Read the model definition and answer for the solid it produces. Units are mm, in the model's axes. A direction names the side the tool comes from. Round coordinates to 2 decimals unless told otherwise and drop trailing zeros.
from build123d import *

# Parameters (mm, degrees)
BOSS_EXTRUDE1_DEPTH     = 15
SKETCH3_W               = 65
SKETCH3_H               = 20
CUT_EXTRUDE2_DEPTH      = 12
CUT_EXTRUDE4_DEPTH      = 52.35659646
M2_TAPPED_HOLE1_D       = 1.6
M2_TAPPED_HOLE1_DEPTH   = 4.519311505
M2_TAPPED_HOLE1_TIP     = 0.480688495
FILLET4_R               = 2.5
SKETCH15_R              = 3
CUT_EXTRUDE10_DEPTH     = 2
CUT_EXTRUDE11_DEPTH     = 8
CUT_EXTRUDE12_DEPTH     = 10
CUT_EXTRUDE13_DEPTH     = 10
SKETCH19_W              = 0.9966679
SKETCH19_H              = 1.5
BOSS_EXTRUDE2_DEPTH     = 20
LPATTERN1_COUNT         = 4
LPATTERN1_PITCH         = 5.5
MIRROR2_COPY_1_SKETCH_W = 0.9966679
MIRROR2_COPY_1_SKETCH_H = 1.5
MIRROR2_COPY_1_DEPTH    = 20
MIRROR2_COPY_2_SKETCH_W = 0.9966679
MIRROR2_COPY_2_SKETCH_H = 1.5
MIRROR2_COPY_2_DEPTH    = 20
MIRROR2_COPY_3_SKETCH_W = 0.9966679
MIRROR2_COPY_3_SKETCH_H = 1.5
MIRROR2_COPY_3_DEPTH    = 20
SKETCH20_W              = 2
SKETCH20_H              = 6
CUT_EXTRUDE14_DEPTH     = 6.5


with BuildPart() as part:
    # Sketch1 → Boss-Extrude1 (new body)
    with BuildSketch(Plane(origin=(0, 0, 0), x_dir=(1, 0, 0), z_dir=(0, 1, 0))):
        Polygon((-47.5, -6.5), (-41.5, -12.5), (41.5, -12.5), (47.5, -6.5), (47.5, 6.5), (41.5, 12.5), (-41.5, 12.5), (-47.5, 6.5), align=None)
    extrude(amount=BOSS_EXTRUDE1_DEPTH)

    # Sketch3 → Cut-Extrude2 (cut)
    with BuildSketch(Plane(origin=(0, 15, 0), x_dir=(1, 0, 0), z_dir=(0, 1, 0))):
        Rectangle(SKETCH3_W, SKETCH3_H)
    extrude(amount=-CUT_EXTRUDE2_DEPTH, mode=Mode.SUBTRACT)

    # Sketch4 → Cut-Extrude4 (cut, through all)
    with BuildSketch(Plane(origin=(0, 15, 0), x_dir=(1, 0, 0), z_dir=(0, 1, 0))):
        with BuildLine():
            Line((41.610912703, 9.560660172), (45.696699141, 5.474873734))
            ThreePointArc((45.696699141, 5.474873734), (45.98959236, 4.767766953), (45.696699141, 4.060660172))
            Line((45.696699141, 4.060660172), (43.575378798, 1.939339828))
            ThreePointArc((43.575378798, 1.939339828), (42.868272016, 1.646446609), (42.161165235, 1.939339828))
            Line((42.161165235, 1.939339828), (38.075378798, 6.025126266))
            ThreePointArc((38.075378798, 6.025126266), (37.782485579, 6.732233047), (38.075378798, 7.439339828))
            Line((38.075378798, 7.439339828), (40.196699141, 9.560660172))
            ThreePointArc((40.196699141, 9.560660172), (40.903805922, 9.853553391), (41.610912703, 9.560660172))
        make_face()
    extrude(amount=-CUT_EXTRUDE4_DEPTH, mode=Mode.SUBTRACT)

    # M2 Tapped Hole1
    with Locations(Plane(origin=(-36.5, 15, 7), x_dir=(0, 0, 1), z_dir=(0, 1, 0))):
        with Locations((0, 0), (-14, 0), (-7, 73)):
            Hole(M2_TAPPED_HOLE1_D / 2, depth=M2_TAPPED_HOLE1_DEPTH)
            with Locations((0, 0, -(M2_TAPPED_HOLE1_DEPTH + M2_TAPPED_HOLE1_TIP / 2))):  # 118° drill point
                Cone(0, M2_TAPPED_HOLE1_D / 2, M2_TAPPED_HOLE1_TIP, mode=Mode.SUBTRACT)

    # Fillet4
    fillet4_edges = [part.edges().sort_by_distance(p)[0] for p in [
        (-47.5, 7.5, -6.5),
        (-41.5, 7.5, -12.5),
        (41.5, 7.5, -12.5),
        (47.5, 7.5, -6.5),
        (47.5, 7.5, 6.5),
        (41.5, 7.5, 12.5),
        (-41.5, 7.5, 12.5),
        (-47.5, 7.5, 6.5),
    ]]
    fillet(fillet4_edges, radius=FILLET4_R)

    # Sketch15 → Cut-Extrude10 (cut)
    with BuildSketch(Plane.XY.offset(-10)):
        with Locations((0, 8.884553107)):
            Circle(SKETCH15_R)
    extrude(amount=-CUT_EXTRUDE10_DEPTH, mode=Mode.SUBTRACT)

    # Sketch16 → Cut-Extrude11 (cut)
    with BuildSketch(Plane.ZY.offset(47.5)):
        Polygon((0, 10.1), (-2.25166605, 8.8), (-2.25166605, 6.2), (0, 4.9), (2.25166605, 6.2), (2.25166605, 8.8), align=None)
    extrude(amount=-CUT_EXTRUDE11_DEPTH, mode=Mode.SUBTRACT)

    # Sketch5 → Cut-Extrude12 (cut)
    with BuildSketch(Plane(origin=(27, 0, 27), x_dir=(0.7071067811865469, 0, -0.7071067811865481), z_dir=(0.7071067811865481, 0, 0.7071067811865469))):
        Polygon((24.748737342, 8.2), (22.497071292, 6.9), (22.497071292, 4.3), (24.748737342, 3), (27.000403391, 4.3), (27.000403391, 6.9), align=None)
    extrude(amount=-CUT_EXTRUDE12_DEPTH, mode=Mode.SUBTRACT)

    # Sketch17 → Cut-Extrude13 (cut)
    with BuildSketch(Plane.XY.offset(12.5)):
        Polygon((8.24833395, 7.3), (7.25166605, 7.3), (5, 8.6), (2.74833395, 7.3), (2.74833395, 4.7), (5, 3.4), (7.25166605, 4.7), (8.24833395, 4.7), (10.5, 3.4), (12.75166605, 4.7), (13.74833395, 4.7), (16, 3.4), (18.25166605, 4.7), (19.24833395, 4.7), (21.5, 3.4), (23.75166605, 4.7), (24.74833395, 4.7), (27, 3.4), (29.25166605, 4.7), (29.25166605, 7.3), (27, 8.6), (24.74833395, 7.3), (23.75166605, 7.3), (21.5, 8.6), (19.24833395, 7.3), (18.25166605, 7.3), (16, 8.6), (13.74833395, 7.3), (12.75166605, 7.3), (10.5, 8.6), align=None)
    cut_extrude13 = extrude(amount=-CUT_EXTRUDE13_DEPTH, mode=Mode.SUBTRACT)

    # Mirror1: Cut-Extrude13 across plane
    add(cut_extrude13.mirror(Plane(origin=(0, 0, 0), x_dir=(0, 0, 1), z_dir=(1, 0, 0))), mode=Mode.SUBTRACT)

    # Sketch19 → Boss-Extrude2 (add)
    with BuildSketch(Plane(origin=(0, 0, 10), x_dir=(-1, 0, 0), z_dir=(0, 0, -1))):
        with Locations((-24.25, 3.75)):
            Rectangle(SKETCH19_W, SKETCH19_H)
    boss_extrude2 = extrude(amount=BOSS_EXTRUDE2_DEPTH)

    # LPattern1: Boss-Extrude2 ×4
    with Locations(*[(-i * LPATTERN1_PITCH, 0, 0) for i in range(1, LPATTERN1_COUNT)]):
        add(boss_extrude2)

    # Mirror2: Boss-Extrude2 across plane
    add(boss_extrude2.mirror(Plane(origin=(0, 0, 0), x_dir=(0, 0, 1), z_dir=(1, 0, 0))))

    # Mirror2 copy 1 sketch → Mirror2 copy 1 (add)
    with BuildSketch(Plane(origin=(5.5, 0, 10), x_dir=(1, 0, 0), z_dir=(0, 0, -1))):
        with Locations((-24.25, -3.75)):
            Rectangle(MIRROR2_COPY_1_SKETCH_W, MIRROR2_COPY_1_SKETCH_H)
    extrude(amount=MIRROR2_COPY_1_DEPTH)

    # Mirror2 copy 2 sketch → Mirror2 copy 2 (add)
    with BuildSketch(Plane(origin=(11, 0, 10), x_dir=(1, 0, 0), z_dir=(0, 0, -1))):
        with Locations((-24.25, -3.75)):
            Rectangle(MIRROR2_COPY_2_SKETCH_W, MIRROR2_COPY_2_SKETCH_H)
    extrude(amount=MIRROR2_COPY_2_DEPTH)

    # Mirror2 copy 3 sketch → Mirror2 copy 3 (add)
    with BuildSketch(Plane(origin=(16.5, 0, 10), x_dir=(1, 0, 0), z_dir=(0, 0, -1))):
        with Locations((-24.25, -3.75)):
            Rectangle(MIRROR2_COPY_3_SKETCH_W, MIRROR2_COPY_3_SKETCH_H)
    extrude(amount=MIRROR2_COPY_3_DEPTH)

    # Sketch20 → Cut-Extrude14 (cut)
    with BuildSketch(Plane(origin=(0, 15, 0), x_dir=(1, 0, 0), z_dir=(0, 1, 0))):
        Polygon((39.364466094, -8.407106781), (37.950252532, -6.992893219), (42.192893219, -2.750252532), (43.607106781, -4.164466094), align=None)
        with Locations((-36.5, 0)):
            Rectangle(SKETCH20_W, SKETCH20_H)
    extrude(amount=-CUT_EXTRUDE14_DEPTH, mode=Mode.SUBTRACT)


solid = part.part
Q1. Straight lines are drawn through the part: probe 1 along X at (y, z) = (12.7, 0); probe 2 along Z at (x, y) = (21, 13); probe 3 along X at (y, z) = (13.75, -7). For each, find the intervals that lie inside material, in ascending order.
Verdict:
probe 1: x = -47.5 to -37.5, -35.5 to -32.5, 32.5 to 35.7, 37.3 to 47.5
probe 2: z = -12.5 to -10, 10 to 12.5
probe 3: x = -46.97 to -37.3, -35.7 to -32.5, 32.5 to 37.82, 44.17 to 46.97
Q2. Determine the mould class of faces 1 (the flat face through (7.252, 4, 0)), 2 (the flat face through (-22.61, 4.04, 11.27)), 3 (the conical face through (-36.383, 10.083, -6.925)) for opening direction Y: pulls with the +Y half, pulls with the -Y half, needs draft (parallel to the pull), parting line crosses it, or undercut.
Verdict:
face 1: needs draft
face 2: undercut
face 3: pulls with the +Y half
Q3. Section A-A (y = 13.75) is taken. State how many separate pieces and enclosed holes the cut face has, then the cut area to 3 significant figures.
Verdict:
separate pieces: 1
enclosed holes: 7
area: 934 mm2
Q4. Flat-ended cylindrical pins translate along their axes: pin 1 Ø2 at (x, z) = (20.5, 3.5) entering from +Y; pin 2 Ø1.8 at (x, z) = (36.5, 0) entering from -Y; pin 3 Ø5 at (x, z) = (-21.5, 3.5) entering from +Y; pin 4 Ø1.2 at (y, z) = (6, 11.5) entering from +X. Find the tip coordinate at first contact, or state that the pin passes through.
Verdict:
pin 1: stops at y = 3
pin 2: stops at y = 0
pin 3: stops at y = 4.5
pin 4: stops at x = 42.91
Q5. Which of the six approach directions +Z, -Z, +X, -X, +Y, -Y give full straight-line access (tool end or side, diameter ignored) to faces 4 (the flat face through (29, 3, 0)), 5 (the flat face through (43.625, 7.605, -7.546)), 6 (the flat face through (40.207, 3.659, 6.821)), 7 (the flat face through (-43.56, 5.54, 1.11)), 8 (the flat face through (14.86, 4.06, 11.27))?
Verdict:
face 4: +Y
face 5: +Y, -Y
face 6: none
face 7: -X
face 8: +Z
